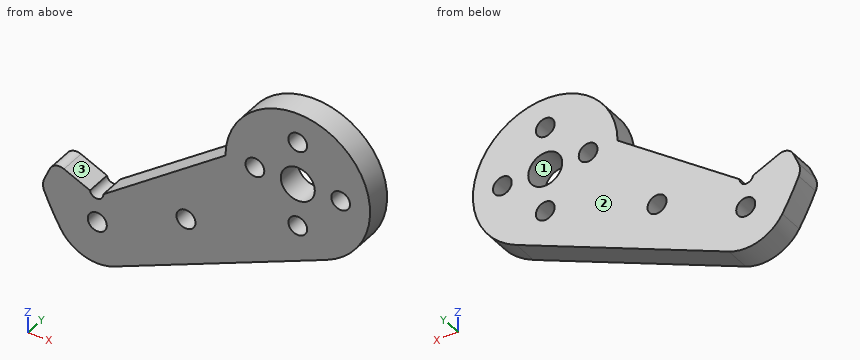
```python
from build123d import *

# Parameters (mm, degrees)
SKETCH1_R           = 1.75
SKETCH1_R_2         = 3.175
SKETCH1_R_3         = 1.778
BOSS_EXTRUDE1_DEPTH = 4.7625


with BuildPart() as part:
    # Sketch1 → Boss-Extrude1 (new body)
    with BuildSketch(Plane(origin=(0, 0, 0), x_dir=(1, 0, 0), z_dir=(0, 1, 0))):
        with BuildLine():
            Line((-38.770225031, 16.757963615), (-43.625448569, 14.598747375))
            ThreePointArc((-43.625448569, 14.598747375), (-45.155674622, 14.559326862), (-46.265582353, 15.613485569))
            Line((-46.265582353, 15.613485569), (-47.282683039, 17.900542834))
            ThreePointArc((-47.282683039, 17.900542834), (-47.541465806, 19.100109045), (-47.298283286, 20.302934833))
            ThreePointArc((-47.298283286, 20.302934833), (-45.865213893, 23.360627542), (-44.234733225, 26.317772344))
            ThreePointArc((-44.234733225, 26.317772344), (-39.855484626, 29.811728531), (-34.259632886, 29.543416329))
            Line((-34.259632886, 29.543416329), (5.363638877, 12.388760148))
            ThreePointArc((5.363638877, 12.388760148), (7.44200849, -11.263503435), (-13.499793526, -0.074664302))
            Line((-13.499793526, -0.074664302), (-36.286855081, 16.495885282))
            ThreePointArc((-36.286855081, 16.495885282), (-37.403602541, 17.810792136), (-38.770225031, 16.757963615))
        make_face()
        with Locations((8, 0)):
            Circle(SKETCH1_R, mode=Mode.SUBTRACT)
        with Locations((0, -8)):
            Circle(SKETCH1_R, mode=Mode.SUBTRACT)
        with Locations((-8, 0)):
            Circle(SKETCH1_R, mode=Mode.SUBTRACT)
        with Locations((0, 8)):
            Circle(SKETCH1_R, mode=Mode.SUBTRACT)
        Circle(SKETCH1_R_2, mode=Mode.SUBTRACT)
        with Locations((-20.862458922, 15.093717491)):
            Circle(SKETCH1_R_3, mode=Mode.SUBTRACT)
        with Locations((-37.413253893, 22.259284205)):
            Circle(SKETCH1_R_3, mode=Mode.SUBTRACT)
    extrude(amount=BOSS_EXTRUDE1_DEPTH)


solid = part.part
```
Design review of the part built by this model. Coordinates are the model's own, in mm. Face numbers are marked on the shaded views. Give positions to 0.01 mm unless a question says otherwise; leave off trailing zeros. Order: outer loops, then holes, each group sorted by start corner. A loop starts at its lowest first (then second) coordinate and runs counter-clockwise, first axis right, second up. Notation, with made-up numbers: M 85.25,5 L 119.25,5 A26 cw 119.25,19 Z; hole C 26,-1.75 d1. An arc over 180 degrees is marked long. One line per question, with ' | ' between items. Start each with the question number.
Q1. We need section B-B (y = 2.8). State how many separate pieces and enclosed holes the cut face has, plus the area to 3 significant figures.
Q2. The part is to be moulded in two halves that separate along Z. For the marked faces 1, 2 and 3, say which applies: +Z half, -Z half, draft (parallel to the pull), parting line (faces both ways), or undercut.
Q3. For L1, parallel to Z at x = 0, y = 1.9 (3 decimals); L2, parallel to X at y = 1.2, z = 0 (3 decimals); L3, parallel to X at y = 0.55, z = -15, list the stretches that pass through material, from the lowest coordinate up. Write a range as [from, to].
Q4. We need section C-C (x = -8). Write out the cut boundary in (y, z), plus the area to 3 significant figures.
Q5. For pin 1 Ø1.5 at (y, z) = (1.5, -10.5) entering from +X; pin 2 Ø2 at (x, y) = (-7, 1.5) entering from -Z, all flat-tipped, find the tip position at first contact; note any pin that passes through.
Q6. We need section A-A (z = -8). Write out the cut boundary in (x, y).
Returned:
1) separate pieces: 1 | enclosed holes: 7 | area: 1,100 mm2
2) face 1: undercut | face 2: draft | face 3: +Z half
3) L1: [-14.711, -9.75], [-6.25, -3.175], [3.175, 6.25], [9.75, 13.5] | L2: [-13.602, -9.75], [-6.25, -3.175], [3.175, 6.25], [9.75, 13.5] | L3: [-45.84, -42.72], [-34.23, -22.64], [-19.09, -0.67]
4) outline: M 0,-18.17 L 4.76,-18.17 L 4.76,-1.75 L 0,-1.75 Z; M 0,1.75 L 4.76,1.75 L 4.76,10.87 L 0,10.87 Z | area: 122 mm2
5) pin 1: x = 9.34 | pin 2: z = -18.17
6) outline: M -24.6,0 L -1.75,0 L -1.75,4.76 L -24.6,4.76 Z; M 1.75,0 L 10.87,0 L 10.87,4.76 L 1.75,4.76 Z
